```python
from build123d import *

# Parameters (mm, degrees)
F0_W     = 25.4
F0_H     = 25.4
F1_DEPTH = 25.4
F5_D     = 3.2639
F5_DEPTH = 7.62
F5_TIP   = 0.9805744872
F6_D     = 3.2639
F6_DEPTH = 7.62
F6_TIP   = 0.9805744872
F7_D     = 3.2639
F7_DEPTH = 7.62
F7_TIP   = 0.9805744872


with BuildPart() as f1:
    # F0 (on Top) → F1 (new body)
    with BuildSketch(Plane.XY):
        Rectangle(F0_W, F0_H)
    extrude(amount=F1_DEPTH)

    # F5
    with Locations(Plane.XY.offset(25.4)):
        with Locations((0, 0)):
            Hole(F5_D / 2, depth=F5_DEPTH)
            with Locations((0, 0, -(F5_DEPTH + F5_TIP / 2))):  # 118° drill point
                Cone(0, F5_D / 2, F5_TIP, mode=Mode.SUBTRACT)

    # F6
    with Locations(Plane.YZ.offset(12.7)):
        with Locations((0, 13.2126277313)):
            Hole(F6_D / 2, depth=F6_DEPTH)
            with Locations((0, 0, -(F6_DEPTH + F6_TIP / 2))):  # 118° drill point
                Cone(0, F6_D / 2, F6_TIP, mode=Mode.SUBTRACT)

    # F7
    with Locations(Plane(origin=(0, 12.7, 0), x_dir=(-1, 0, 0), z_dir=(0, 1, 0))):
        with Locations((0, 11.9171617553)):
            Hole(F7_D / 2, depth=F7_DEPTH)
            with Locations((0, 0, -(F7_DEPTH + F7_TIP / 2))):  # 118° drill point
                Cone(0, F7_D / 2, F7_TIP, mode=Mode.SUBTRACT)


solid = f1.part
```
Verification items for the finished model (mm, model axes). A direction names the side the tool comes from. Coordinates: 2 decimals unless noted, no trailing zeros. Answer as a JSON object with one key per item and string values.
(1) Scan lines: line 1 along Z through (x, y) = (6.75, 0); line 2 along X through (y, z) = (0, 22). Record each from-to range of solid material in increasing order.
Response:
{"line 1": "z = 0 to 11.58, 14.84 to 25.4", "line 2": "x = -12.7 to -1.63, 1.63 to 12.7"}
(2) Go/stop test with a flat-tipped pin: pin 1 Ø8 at (x, y) = (-6.5, -8) entering from -Z. Record where the tip stops, or that it passes through.
Response:
{"pin 1": "stops at z = 0"}
(3) Access from +Z, -Z, +X, -X, +Y, -Y to the whole of each face (thin tool, end or side, straight path). Record for faces 1 (the cylindrical face through (-0.212, 8.837, 13.535)), 2 (the flat face through (12.7, 0, 15)), 3 (the flat face through (0, 0, 0)), 4 (the cylindrical face through (0.354, -1.593, 21.537)), 5 (the cylindrical face through (8.84, 0.35, 11.62)).
Response:
{"face 1": "+Y", "face 2": "+Z, -Z, +X, +Y, -Y", "face 3": "-Z, +X, -X, +Y, -Y", "face 4": "+Z", "face 5": "+X"}
(4) Mould release check, pull along Y, two halves, no side actions. Record for faces 6 (the flat face through (0, -12.7, 13)), 7 (the conical face through (4.27, -0.061, 12.936)), 8 (the flat face through (-12.7, 0, 13)): pulls with the +Y half, pulls with the -Y half, needs draft (parallel to the pull), parting line crosses it, or undercut.
Response:
{"face 6": "pulls with the -Y half", "face 7": "undercut", "face 8": "needs draft"}
